Geometry: final body of the model. Coordinates: model frame, mm. A direction names the side the tool comes from. Coordinates: 2 decimals unless noted, no trailing zeros. Write each loop counter-clockwise with the first axis right and the second up, starting at its lowest first coordinate (ties: lowest second). Pieces come first, ordered by that corner, then holes. Notation, with made-up numbers: (9, 33) -> (46, 33) arc R19 ccw to (46, 44) -> close; hole circle Ø1 at (-10.75, -19.5). An arc over 180 degrees is marked (long way). One line per item, written item: value.
```python
from build123d import *

# Parameters (mm, degrees)
SKETCH1_R           = 9.7536
BOSS_EXTRUDE1_DEPTH = 3.4798


with BuildPart() as part:
    # Sketch1 → Boss-Extrude1 (new body)
    with BuildSketch(Plane(origin=(0, 0, 0), x_dir=(1, 0, 0), z_dir=(0, 1, 0))):
        with Locations(Location((0, 0, 0), (0, 0, 270))):
            Circle(SKETCH1_R)
        with BuildLine():
            ThreePointArc((3.812821178, 6.604), (4.03243642, 6.384384758), (4.112821178, 6.084384758))
            Line((4.112821178, 6.084384758), (7.325642355, 0.519615242))
            ThreePointArc((7.325642355, 0.519615242), (7.545257598, 0.3), (7.625642355, 0))
            ThreePointArc((7.625642355, 0), (7.545257598, -0.3), (7.325642355, -0.519615242))
            Line((7.325642355, -0.519615242), (4.112821178, -6.084384758))
            ThreePointArc((4.112821178, -6.084384758), (4.03243642, -6.384384758), (3.812821178, -6.604))
            ThreePointArc((3.812821178, -6.604), (3.512821178, -6.684384758), (3.212821178, -6.604))
            Line((3.212821178, -6.604), (-3.212821178, -6.604))
            ThreePointArc((-3.212821178, -6.604), (-3.512821178, -6.684384758), (-3.812821178, -6.604))
            ThreePointArc((-3.812821178, -6.604), (-4.03243642, -6.384384758), (-4.112821178, -6.084384758))
            Line((-4.112821178, -6.084384758), (-7.325642355, -0.519615242))
            ThreePointArc((-7.325642355, -0.519615242), (-7.545257598, -0.3), (-7.625642355, 0))
            ThreePointArc((-7.625642355, 0), (-7.545257598, 0.3), (-7.325642355, 0.519615242))
            Line((-7.325642355, 0.519615242), (-4.112821178, 6.084384758))
            ThreePointArc((-4.112821178, 6.084384758), (-4.03243642, 6.384384758), (-3.812821178, 6.604))
            ThreePointArc((-3.812821178, 6.604), (-3.512821178, 6.684384758), (-3.212821178, 6.604))
            Line((-3.212821178, 6.604), (3.212821178, 6.604))
            ThreePointArc((3.212821178, 6.604), (3.512821178, 6.684384758), (3.812821178, 6.604))
        make_face(mode=Mode.SUBTRACT)
    extrude(amount=BOSS_EXTRUDE1_DEPTH)


solid = part.part
```
(1) Section C-C (z = -0.75). Return the cut outline in (x, y).
Responses:
outline: (-9.72, 0) -> (-7.19, 0) -> (-7.19, 3.48) -> (-9.72, 3.48) -> close; (7.19, 0) -> (9.72, 0) -> (9.72, 3.48) -> (7.19, 3.48) -> close
(2) Line query: line 1 (Z direction, x = 1, y = 3); line 2 (Z direction, x = 5.5, y = 2.35); line 3 (X direction, y = 2.9, z = -1.5). Output: solid intervals per line, ascending. Write a range as [from, to].
Responses:
line 1: z = [-9.7, -6.6], [6.6, 9.7]
line 2: z = [-8.05, -3.68], [3.68, 8.05]
line 3: x = [-9.64, -6.76], [6.76, 9.64]
(3) Section B-B (y = 2.4). Return the cut outline in (x, z).
Responses:
outline: circle Ø19.51 at (0, 0); hole (-7.33, -0.52) -> (-4.11, -6.08) arc R0.6 ccw to (-3.21, -6.6) -> (3.21, -6.6) arc R0.6 ccw to (4.11, -6.08) -> (7.33, -0.52) arc R0.6 ccw to (7.33, 0.52) -> (4.11, 6.08) arc R0.6 ccw to (3.21, 6.6) -> (-3.21, 6.6) arc R0.6 ccw to (-4.11, 6.08) -> (-7.33, 0.52) arc R0.6 ccw to start
(4) Section D-D (x = -8). Return the cut outline in (y, z).
Responses:
outline: (0, -5.58) -> (3.48, -5.58) -> (3.48, 5.58) -> (0, 5.58) -> close
(5) Section A-A (x = 0). Return the cut outline in (y, z), then the cut area to 3 significant figures.
Responses:
outline: (0, -9.75) -> (3.48, -9.75) -> (3.48, -6.6) -> (0, -6.6) -> close; (0, 6.6) -> (3.48, 6.6) -> (3.48, 9.75) -> (0, 9.75) -> close
area: 21.9 mm2
(6) Reachability of faces 4 (the flat face through (0, 2, -6.604)), 5 (the flat face through (0, 3.48, -7)) from +Z, -Z, +X, -X, +Y, -Y: full face, straight path, thin tool, end or side. Return the list, or none.
Responses:
face 4: +Y, -Y
face 5: +Z, -Z, +X, -X, +Y
(7) Pull-direction query (X, two-part tool) for faces 1 (the flat face through (5.742, 1.716, 3.263)), 2 (the flat face through (0, 0, -7)), 3 (the cylindrical face through (2.93, 1.716, 9.303)); classes: released by +X, released by -X, zero draft, split by the parting line, or undercut.
Responses:
face 1: undercut
face 2: zero draft
face 3: split by the parting line
